Study the drawing (mm; zero at the part's minimum x, y, z) and answer. Round coordinates to 2 decimals unless told otherwise and drop trailing zeros. Loops run counter-clockwise (first coordinate to the right, second up) from the corner with the lowest first, then second, coordinate; pieces in that order, holes last. Notation, with made-up numbers: (9.25, 51) -> (22.25, 51) arc R36 cw to (22.25, 88) -> close; hole circle Ø11 at (39.25, -5.5). An arc over 180 degrees is marked (long way). Answer in a Markdown table with one row per item. Add a question column.
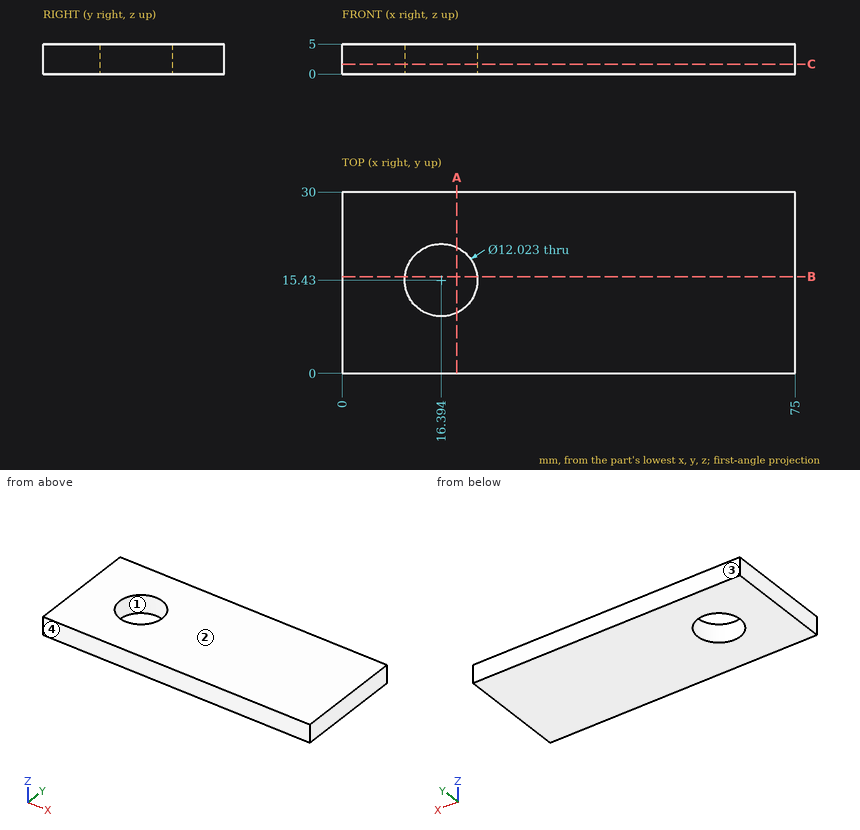
Item 1: Section C-C, the plane z = 1.65 is taken. Write down the section's boundary in (x, y).
Item 2: The mould has two halves that part along Y. Classify the marked faces 1, 2, 3 and 4: +Y half, -Y half, draft (parallel to the pull), parting line (faces both ways), or undercut.
Item 3: A flat-ended cylindrical pin translates along its axis: P1, Ø1, axis at x = 58, y = 19.5, coming from the -Z side. Find the tip coordinate at first contact, or state that the pin passes through.
Item 4: Section B-B, the plane y = 16 is taken. Write down the section's boundary in (x, z).
Item 5: Section A-A, the plane x = 19 is taken. Write down the section's boundary in (y, z), and give its area (3 significant figures).
Item 6: Consider L1, parallel to X at y = 20.25, z = 0.75; L2, parallel to X at y = 17, z = 1.75; L3, parallel to Y at x = 14.5, z = 4.4 (1 decimal). Determine where each line is inside the solid, lowest interval first. Write a range as from..to.
Here are the results:
| question | item | result |
|---|---|---|
| 1 | outline | (0, 0) -> (75, 0) -> (75, 30) -> (0, 30) -> close; hole circle Ø12.02 at (16.39, 15.43) |
| 2 | face 1 | undercut |
| 2 | face 2 | draft |
| 2 | face 3 | +Y half |
| 2 | face 4 | -Y half |
| 3 | P1 | stops at z = 0 |
| 4 | outline | (0, 0) -> (10.41, 0) -> (10.41, 5) -> (0, 5) -> close; (22.38, 0) -> (75, 0) -> (75, 5) -> (22.38, 5) -> close |
| 5 | outline | (0, 0) -> (10.01, 0) -> (10.01, 5) -> (0, 5) -> close; (20.85, 0) -> (30, 0) -> (30, 5) -> (20.85, 5) -> close |
| 5 | area | 95.8 mm² |
| 6 | L1 | x = 0..12.8, 19.99..75 |
| 6 | L2 | x = 0..10.59, 22.2..75 |
| 6 | L3 | y = 0..9.7, 21.1..30 |
